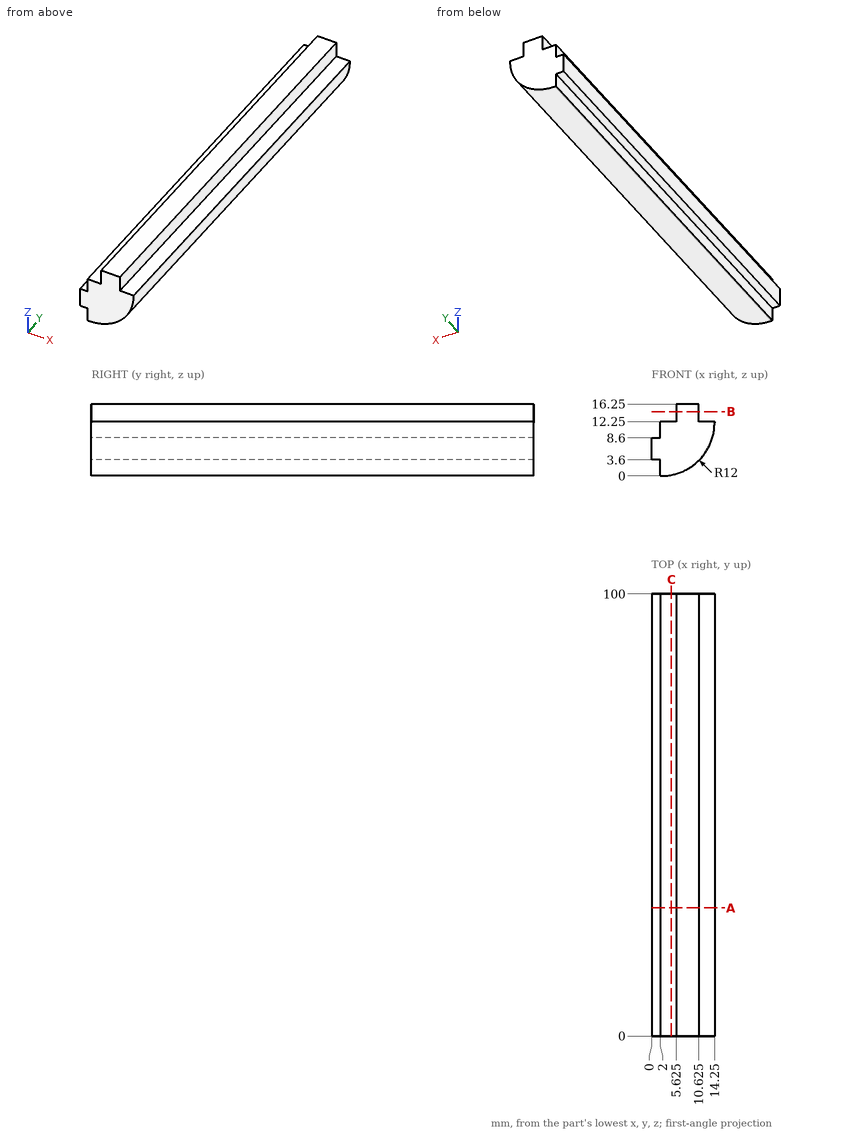
The figure shows three views and two pictorial views of one solid part (mm, origin at its lowest corner). Answer the questions. Coordinates: 2 decimals unless noted, no trailing zeros. Loops run counter-clockwise (first coordinate to the right, second up) from the corner with the lowest first, then second, coordinate; pieces in that order, holes last.
(1) The part is cut by section C-C (x = 4.5). Determine the outline of the cut face in (y, z), and give its area (3 significant figures).
Solution:
outline: (0, 0.21) - (100, 0.21) - (100, 12.25) - (0, 12.25) - close
area: 1,200 mm2
(2) Consider line 1 along X through (y, z) = (64, 11.75); line 2 along X through (y, z) = (85, 12.75) (3 decimals); line 3 along Z through (x, y) = (2.5, 21). Determine where each line is inside the solid, lowest interval first.
Solution:
line 1: x = 2 to 14.25
line 2: x = 5.625 to 10.625
line 3: z = 0 to 12.25
(3) The part is cut by section B-B (z = 14.5). Determine the outline of the cut face in (x, y) (3 decimals), and give its area (3 significant figures).
Solution:
outline: (5.625, 0) - (10.625, 0) - (10.625, 100) - (5.625, 100) - close
area: 500 mm2
(4) The part is cut by section A-A (y = 29). Determine the outline of the cut face in (x, z) (3 decimals), and give its area (3 significant figures).
Solution:
outline: (0, 3.6) - (2, 3.6) - (2, 0) - (2.25, 0) arc R12 ccw to (14.25, 12) - (14.25, 12.25) - (10.625, 12.25) - (10.625, 16.25) - (5.625, 16.25) - (5.625, 12.25) - (2, 12.25) - (2, 8.6) - (0, 8.6) - close
area: 149 mm2
(5) Flat-ended cylindrical pins translate along their axes: pin 1 Ø3 at (y, z) = (35.5, 13.5) entering from +X; pin 2 Ø6 at (y, z) = (43, 3) entering from +X; pin 3 Ø1.8 at (x, y) = (12, 32) entering from +Z; pin 4 Ø1.1 at (y, z) = (64.5, 1.5) entering from -X. Find the tip coordinate at first contact, or state that the pin passes through.
Solution:
pin 1: stops at x = 14.25
pin 2: stops at x = 12.64
pin 3: stops at z = 12.25
pin 4: stops at x = 2
